Design review of the part built by this model. Coordinates are the model's own, in mm. Coordinates: 2 decimals unless noted, no trailing zeros. Loops run counter-clockwise (first coordinate to the right, second up) from the corner with the lowest first, then second, coordinate; pieces in that order, holes last. Notation, with made-up numbers: (-35, 28.25) - (-19, 28.25) arc R30 ccw to (-19, 58.25) - close; hole circle Ø3 at (48.25, -12). An arc over 180 degrees is marked (long way). Use one line per item in the form item = value. Start each with the question number.
(1) For L1, parallel to X at y = 5.75, z = 58; L2, parallel to Z at x = -8.5, y = 3.5; L3, parallel to Z at x = -23, y = 2.25, list the stretches that pass through material, from the lowest coordinate up.
(2) Add section B-B (z = 58). State the section outline as (x, y) points, plus the area to 3 significant figures.
(3) Add section C-C (y = 6.25). State the section outline as (x, z) points, plus the area to 3 significant figures.
(4) Add section D-D (z = 79.5). State the section outline as (x, y) points.
(5) Clearance check with flat-ended pins moving along their axes: pin 1 Ø2 at (x, y) = (-34.5, 1) entering from +Z; pin 2 Ø1.5 at (x, y) = (-42.5, 4.5) entering from -Z; pin 3 Ø7 at (x, z) = (17, 58) entering from +Y. State where each tip first meets the part, or that it passes through.
(6) Add section A-A (x = 17). State the section outline as (y, z) points.
```python
from build123d import *

# Parameters (mm, degrees)
SKETCH1_R           = 33
SKETCH1_R_2         = 4.5
BOSS_EXTRUDE1_DEPTH = 7.8


with BuildPart() as part:
    # Sketch1 → Boss-Extrude1 (new body)
    with BuildSketch(Plane(origin=(0, 0, 0), x_dir=(1, 0, 0), z_dir=(0, 1, 0))):
        with BuildLine():
            Line((0, 0), (36, 0))
            Line((36, 0), (36, -116))
            Line((36, -116), (0, -116))
            ThreePointArc((0, -116), (-58, -58), (0, 0))
        make_face()
        with Locations(Location((-22, -58, 0), (0, 0, 270))):
            Circle(SKETCH1_R, mode=Mode.SUBTRACT)
        with Locations(Location((17, -58, 0), (0, 0, 270))):
            Circle(SKETCH1_R_2, mode=Mode.SUBTRACT)
    extrude(amount=BOSS_EXTRUDE1_DEPTH)


solid = part.part
```
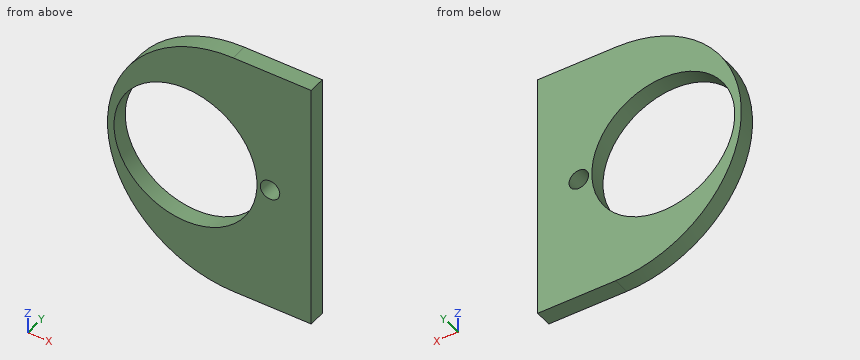
Computed values:
q1.L1 = -58 to -55, 11 to 12.5, 21.5 to 36
q1.L2 = 0.63 to 27.89, 88.11 to 115.37
q1.L3 = 4.76 to 25.02, 90.98 to 111.24
q2.outline = (-58, 0) - (-55, 0) - (-55, 7.8) - (-58, 7.8) - close; (11, 0) - (12.5, 0) - (12.5, 7.8) - (11, 7.8) - close; (21.5, 0) - (36, 0) - (36, 7.8) - (21.5, 7.8) - close
q2.area = 148 mm^2
q3.outline = (0, 0) - (36, 0) - (36, 116) - (0, 116) arc R58 ccw to start; hole circle Ø66 at (-22, 58); hole circle Ø9 at (17, 58)
q3.area = 5,980 mm^2
q4.outline = (-53.87, 0) - (-47.03, 0) - (-47.03, 7.8) - (-53.87, 7.8) - close; (3.03, 0) - (36, 0) - (36, 7.8) - (3.03, 7.8) - close
q5.pin_1 = 105.35
q5.pin_2 = 17.74
q5.pin_3 = through
q6.outline = (0, 0) - (7.8, 0) - (7.8, 53.5) - (0, 53.5) - close; (0, 62.5) - (7.8, 62.5) - (7.8, 116) - (0, 116) - close
